Design review of the part built by this model. Coordinates are the model's own, in mm. A direction names the side the tool comes from. Round coordinates to 2 decimals unless told otherwise and drop trailing zeros. Loops run counter-clockwise (first coordinate to the right, second up) from the corner with the lowest first, then second, coordinate; pieces in that order, holes last. Notation, with made-up numbers: (-18, 14.5) - (-10, 14.5) arc R22 cw to (-10, 21.5) - close; hole circle Ø9 at (-27, 24.25). An arc over 180 degrees is marked (long way). Answer as CSV lines item,"result". Start each with the question number.
(1) Consider section C-C (z = 8). Give the boundary of the cut face in (x, y).
(2) For faces 1 (the flat face through (0, 15, 10)), 2 (the flat face through (6, 29, 20)), 3 (the flat face through (10, 30, 10)), list the 3-axis set-ups (+Z, -Z, +X, -X, +Y, -Y) from which the entire face can be reached by the end or side of a thin tool; tool diameter is ignored.
(3) Consider section B-B (x = 15). Give the boundary of the cut face in (y, z).
(4) Consider section D-D (y = 14). Give the boundary of the cut face in (x, z).
(5) Consider section A-A (y = 32.5). Give the boundary of the cut face in (x, z), and give its area (3 significant figures).
(6) For P1, Ø12, axis at y = 31, z = 30.5, coming from the +X side; P2, Ø10, axis at x = 12, y = 13, coming from the +Z side; P3, Ø2, axis at y = 12, z = 34, coming from the -X side; P4, Ø3, axis at x = 34, y = 33, coming from the +Z side, all flat-tipped, find the tip position at first contact; note any pin that passes through.
(7) Wall thickness on L1, parallel to X at y = 36.5, z = 6.5; L2, parallel to Z at x = 8.5, y = 4.5; L3, parallel to X at y = 13.5, z = 31.5: over which ranges is each line inside the solid? List them lowest first.
from build123d import *

# Parameters (mm, degrees)
SKETCH1_W           = 40
SKETCH1_H           = 40
BOSS_EXTRUDE1_DEPTH = 40
CUT_EXTRUDE1_DEPTH  = 40
CUT_EXTRUDE2_DEPTH  = 40
CUT_EXTRUDE3_DEPTH  = 20
CUT_EXTRUDE4_DEPTH  = 20
CUT_EXTRUDE7_DEPTH  = 49


with BuildPart() as part:
    # Sketch1 → Boss-Extrude1 (new body)
    with BuildSketch(Plane.XY):
        with Locations((20, 20)):
            Rectangle(SKETCH1_W, SKETCH1_H)
    extrude(amount=BOSS_EXTRUDE1_DEPTH)

    # Sketch2 → Cut-Extrude1 (cut)
    with BuildSketch(Plane.ZY):
        Polygon((40, 0), (20, 40), (40, 40), align=None)
    extrude(amount=-CUT_EXTRUDE1_DEPTH, mode=Mode.SUBTRACT)

    # Sketch3 → Cut-Extrude2 (cut)
    with BuildSketch(Plane.XZ):
        Polygon((0, 20), (20, 40), (0, 40), align=None)
    extrude(amount=-CUT_EXTRUDE2_DEPTH, mode=Mode.SUBTRACT)

    # Sketch4 → Cut-Extrude3 (cut)
    with BuildSketch(Plane.ZY):
        Polygon((20, 40), (0, 20), (0, 40), align=None)
    extrude(amount=-CUT_EXTRUDE3_DEPTH, mode=Mode.SUBTRACT)

    # Sketch5 → Cut-Extrude4 (cut)
    with BuildSketch(Plane(origin=(-8.888888889, 4.444444444, 8.888888889), x_dir=(0.745355992, 0.298142397, 0.596284794), z_dir=(-0.666666667, 0.333333333, 0.666666667))):
        Polygon((38.75851161, 26.83281573), (38.75851161, -17.88854382), (11.92569588, -8.94427191), align=None)
    extrude(amount=CUT_EXTRUDE4_DEPTH, mode=Mode.SUBTRACT)

    # Sketch8 → Cut-Extrude7 (cut)
    with BuildSketch(Plane.XY.offset(20)):
        Polygon((20, 40), (0, 0), (0, 40), align=None)
    extrude(amount=CUT_EXTRUDE7_DEPTH, mode=Mode.SUBTRACT)


solid = part.part
Determined:
1,outline,"(0, 0) - (40, 0) - (40, 40) - (20, 40) - (20, 28) - (0, 28) - close"
2,face 1,"+Z, -Z, -X, +Y, -Y"
2,face 2,"+Z, -X, +Y"
2,face 3,"-Z, -X, +Y"
3,outline,"(0, 0) - (20, 0) - (40, 20) - (30, 20) - (0, 35) - close"
4,outline,"(0, 0) - (40, 0) - (40, 33) - (20, 33) - (7, 20) - (0, 20) - close"
5,outline,"(0, 12.5) - (20, 12.5) - (20, 0) - (40, 0) - (40, 23.75) - (20, 23.75) - (16.25, 20) - (0, 20) - close"
5,area,"632 mm^2"
6,P1,"stops at x = 40"
6,P2,"stops at z = 31.09"
6,P3,"stops at x = 18.88"
6,P4,"stops at z = 24.25"
7,L1,"x = 20 to 40"
7,L2,"z = 0 to 26.25"
7,L3,"x = 18.25 to 40"
